Model file for the job. Use its own axes, mm. A direction names the side the tool comes from. Round coordinates to 2 decimals unless told otherwise and drop trailing zeros. Order: outer loops, then holes, each group sorted by start corner. A loop starts at its lowest first (then second) coordinate and runs counter-clockwise, first axis right, second up. Notation, with made-up numbers: (12, -37.75) -> (49, -37.75) arc R15 cw to (49, -33.75) -> close; hole circle Ø10 at (62, 48). An arc over 180 degrees is marked (long way). Put each result on its own line as item: value. Start each with the question number.
Q1. Cut at A-A, the plane x = 3.85. List the corners of the cut face in (y, z), and give its area (3 significant figures).
Q2. Cut at C-C, the plane x = 9.65. List the corners of the cut face in (y, z).
Q3. Flat gauge pin, fed straight in: P1, Ø5.5, axis at x = 3.85, y = -15.5, coming from the +Z side. Where does the tip first touch, or does it go through?
Q4. 3-axis set-ups, long thin cutter, end or side, ignore diameter. For faces 1 (the face through (0, 25, 25)), 2 (the face through (22, 12.6, 31)), 3 (the face through (-10.233, 15, 31)): which of +Z, -Z, +X, -X, +Y, -Y reach the whole face in a straight line?
Q5. Pull direction X, two halves, no side cores. Call faces 4 (the face through (11.988, -15, 31)), 5 (the face through (8.102, 19.019, 1.774)), 6 (the face through (-22, -12.6, 31)): released by +X, released by -X, zero draft, split by the parting line, or undercut.
Q6. Cut at B-B, the plane y = -15.5. List the corners of the cut face in (x, z).
Q7. Cut at D-D, the plane z = 5.5. List the corners of the cut face in (x, y), and give its area (3 significant figures).
Q8. Probe L1, parallel to X at y = 17.6, z = 28; L2, parallel to X at y = -13, z = 32; L3, parallel to Y at x = 9.65, z = 1.1. List the from-to ranges inside material, lowest first.
from build123d import *

# Parameters (mm, degrees)
SKETCH1_W           = 50
SKETCH1_H           = 46.5
BOSS_EXTRUDE1_DEPTH = 11
SKETCH2_W           = 46.5
SKETCH2_H           = 12.4
BOSS_EXTRUDE2_DEPTH = 40
SKETCH3_W           = 5.4
SKETCH3_H           = 5.4
SKETCH3_W_2         = 22.221144714
CUT_EXTRUDE1_DEPTH  = 40
SKETCH4_R           = 4.5
CUT_EXTRUDE2_DEPTH  = 47.5
SKETCH5_R           = 2.1
CUT_EXTRUDE3_DEPTH  = 59.496260564


with BuildPart() as part:
    # Sketch1 → Boss-Extrude1 (new body)
    with BuildSketch(Plane(origin=(0, 0, 0), x_dir=(0, 1, 0), z_dir=(0, 0, 1))):
        Rectangle(SKETCH1_W, SKETCH1_H)
    extrude(amount=BOSS_EXTRUDE1_DEPTH)

    # Sketch2 → Boss-Extrude2 (add)
    with BuildSketch(Plane.XY.offset(11)):
        with Locations((0, 18.8)):
            Rectangle(SKETCH2_W, SKETCH2_H)
        with Locations((0, -18.8)):
            Rectangle(SKETCH2_W, SKETCH2_H)
    extrude(amount=BOSS_EXTRUDE2_DEPTH)

    # Sketch3 → Cut-Extrude1 (cut)
    with BuildSketch(Plane.XY.offset(51)):
        with Locations((-18.35, -15.3)):
            Rectangle(SKETCH3_W, SKETCH3_H)
        with Locations((18.65, -15.3)):
            Rectangle(SKETCH3_W, SKETCH3_H)
        with Locations((18.65, 15.3)):
            Rectangle(SKETCH3_W, SKETCH3_H)
        with Locations((-18.35, 15.3)):
            Rectangle(SKETCH3_W, SKETCH3_H)
        with Locations((0.877150449, 15.3)):
            Rectangle(SKETCH3_W_2, SKETCH3_H)
        with Locations((0.877150449, -15.3)):
            Rectangle(SKETCH3_W_2, SKETCH3_H)
    extrude(amount=-CUT_EXTRUDE1_DEPTH, mode=Mode.SUBTRACT)

    # Sketch4 → Cut-Extrude2 (cut)
    with BuildSketch(Plane.XY.offset(51)):
        with Locations((9.65, 17.6)):
            Circle(SKETCH4_R)
        with Locations((3.85, -15.5)):
            Circle(SKETCH4_R)
    extrude(amount=-CUT_EXTRUDE2_DEPTH, mode=Mode.SUBTRACT)

    # Sketch5 → Cut-Extrude3 (cut, through all)
    with BuildSketch(Plane.XY.offset(3.5)):
        with Locations((3.85, -15.5)):
            Circle(SKETCH5_R)
        with Locations((9.65, 17.6)):
            Circle(SKETCH5_R)
    extrude(amount=-CUT_EXTRUDE3_DEPTH, mode=Mode.SUBTRACT)


solid = part.part
Ans:
1. outline: (-25, 0) -> (-17.6, 0) -> (-17.6, 3.5) -> (-20, 3.5) -> (-20, 51) -> (-25, 51) -> close; (-13.4, 0) -> (25, 0) -> (25, 51) -> (18, 51) -> (18, 11) -> (-11, 11) -> (-11, 3.5) -> (-13.4, 3.5) -> close
1. area: 948 mm^2
2. outline: (-25, 0) -> (15.5, 0) -> (15.5, 3.5) -> (13.1, 3.5) -> (13.1, 11) -> (-18, 11) -> (-18, 51) -> (-25, 51) -> close; (19.7, 0) -> (25, 0) -> (25, 51) -> (22.1, 51) -> (22.1, 3.5) -> (19.7, 3.5) -> close
3. P1: stops at z = 3.5
4. face 1: +Z, -Z, +X, -X, +Y
4. face 2: +Z, +X, -X
4. face 3: +Z
5. face 4: undercut
5. face 5: undercut
5. face 6: zero draft
6. outline: (-23.25, 0) -> (1.75, 0) -> (1.75, 3.5) -> (-0.65, 3.5) -> (-0.65, 11) -> (-10.23, 11) -> (-10.23, 51) -> (-15.65, 51) -> (-15.65, 11) -> (-21.05, 11) -> (-21.05, 51) -> (-23.25, 51) -> close; (5.95, 0) -> (23.25, 0) -> (23.25, 51) -> (21.35, 51) -> (21.35, 11) -> (15.95, 11) -> (15.95, 51) -> (11.99, 51) -> (11.99, 11) -> (8.35, 11) -> (8.35, 3.5) -> (5.95, 3.5) -> close
7. outline: (-23.25, -25) -> (23.25, -25) -> (23.25, 25) -> (-23.25, 25) -> close; hole circle Ø9 at (3.85, -15.5); hole circle Ø9 at (9.65, 17.6)
7. area: 2,200 mm^2
8. L1: x = -23.25 to -21.05, -15.65 to -10.23, 14.15 to 15.95, 21.35 to 23.25
8. L2: x = -23.25 to -21.05, -15.65 to -10.23, 11.99 to 15.95, 21.35 to 23.25
8. L3: y = -25 to 15.5, 19.7 to 25
